```python
from build123d import *

# Parameters (mm, degrees)
SKETCH1_W                     = 96
SKETCH1_H                     = 96
SKETCH1_R                     = 13.97
BOSS_EXTRUDE1_DEPTH           = 5
FILLET1_R                     = 20
CBORE_FOR_M3_SHCS1_AT_2_COUNT = 2
CBORE_FOR_M3_SHCS1_AT_2_PITCH = 56.568542495
CBORE_FOR_M3_SHCS1_AT_3_COUNT = 2
CBORE_FOR_M3_SHCS1_AT_3_PITCH = 80
CBORE_FOR_M3_SHCS1_AT_4_COUNT = 2
CBORE_FOR_M3_SHCS1_AT_4_PITCH = 56.568542495
SKETCH7_R                     = 2
CUT_EXTRUDE1_DEPTH            = 69.066144301


with BuildPart() as part:
    # Sketch1 → Boss-Extrude1 (new body)
    with BuildSketch(Plane(origin=(0, 0, 0), x_dir=(1, 0, 0), z_dir=(0, 1, 0))):
        Rectangle(SKETCH1_W, SKETCH1_H)
        with Locations(Location((0, 0, 0), (0, 0, 270))):
            Circle(SKETCH1_R, mode=Mode.SUBTRACT)
    extrude(amount=BOSS_EXTRUDE1_DEPTH)

    # Fillet1
    fillet1_edges = [part.edges().sort_by_distance(p)[0] for p in [
        (-48, 2.5, -48),
        (48, 2.5, -48),
        (48, 2.5, 48),
        (-48, 2.5, 48),
    ]]
    fillet(fillet1_edges, radius=FILLET1_R)

    # Sketch6 → CBORE for M3 SHCS1 (revolve, cut)
    with BuildSketch(Plane(origin=(-40, 0, 0), x_dir=(0, 0, -1), z_dir=(1, 0, 0))):
        Polygon((0, 0), (0, 5), (1.7, 5), (1.7, 3), (3.25, 3), (3.25, 0.025), (3.275, 0), align=None)
    cbore_for_m3_shcs1 = revolve(axis=Axis((-40, -6.35, 0), (0, 1, 0)), mode=Mode.SUBTRACT)

    # CBORE for M3 SHCS1 at 2: CBORE for M3 SHCS1 ×2
    with Locations(*[Vector(0.7071067811865476, 0, 0.7071067811865476) * (i * CBORE_FOR_M3_SHCS1_AT_2_PITCH) for i in range(1, CBORE_FOR_M3_SHCS1_AT_2_COUNT)]):
        add(cbore_for_m3_shcs1, mode=Mode.SUBTRACT)

    # CBORE for M3 SHCS1 at 3: CBORE for M3 SHCS1 ×2
    with Locations(*[(i * CBORE_FOR_M3_SHCS1_AT_3_PITCH, 0, 0) for i in range(1, CBORE_FOR_M3_SHCS1_AT_3_COUNT)]):
        add(cbore_for_m3_shcs1, mode=Mode.SUBTRACT)

    # CBORE for M3 SHCS1 at 4: CBORE for M3 SHCS1 ×2
    with Locations(*[Vector(0.7071067811865476, 0, -0.7071067811865476) * (i * CBORE_FOR_M3_SHCS1_AT_4_PITCH) for i in range(1, CBORE_FOR_M3_SHCS1_AT_4_COUNT)]):
        add(cbore_for_m3_shcs1, mode=Mode.SUBTRACT)

    # Sketch7 → Cut-Extrude1 (cut, through all)
    with BuildSketch(Plane.XZ):
        with Locations(Location((-27.5, 0, 0), (0, 0, 270))):
            Circle(SKETCH7_R)
        with Locations(Location((0, 27.5, 0), (0, 0, 270))):
            Circle(SKETCH7_R)
        with Locations(Location((27.5, 0, 0), (0, 0, 270))):
            Circle(SKETCH7_R)
        with Locations(Location((0, -27.5, 0), (0, 0, 270))):
            Circle(SKETCH7_R)
    extrude(amount=-CUT_EXTRUDE1_DEPTH, mode=Mode.SUBTRACT)


solid = part.part
```
The model under review builds one solid part; all positions refer to its coordinate system, in mm. A direction names the side the tool comes from. Round coordinates to 2 decimals unless told otherwise and drop trailing zeros. Loops run counter-clockwise (first coordinate to the right, second up) from the corner with the lowest first, then second, coordinate; pieces in that order, holes last. Notation, with made-up numbers: M 28,62 L 51,62 A19 ccw 51,87 Z; hole C -5,38 d4. An arc over 180 degrees is marked long. Put each result on its own line as item: value.
Q1. Consider section A-A, the plane y = 1.7. Count the separate pieces of the cut face and the enclosed holes in it, then the cut area to 3 significant figures.
Result set:
separate pieces: 1
enclosed holes: 9
area: 8,080 mm²
Q2. Mouldability with a two-part tool opening along Z and no side actions: class faces 3 (the cylindrical face through (-0.766, 2.465, 25.653)), 4 (the flat face through (0, 2, -48)), 5 (the cylindrical face through (-42.297, 2.535, 41.986)) as released by +Z, released by -Z, zero draft, split by the parting line, or undercut.
Result set:
face 3: undercut
face 4: released by -Z
face 5: released by +Z
Q3. Consider section D-D, the plane x = -34.5. Give the boundary of the cut face in (y, z), then the cut area to 3 significant figures.
Result set:
outline: M 0,-46.91 L 5,-46.91 L 5,46.91 L 0,46.91 Z
area: 469 mm²
Q4. Consider section B-B, the plane z = -40. Give the boundary of the cut face in (x, y) (3 decimals), then the cut area to 3 significant figures.
Result set:
outline: M -44,0 L -3.275,0 L -3.25,0.025 L -3.25,3 L -1.7,3 L -1.7,5 L -44,5 Z; M 1.7,3 L 3.25,3 L 3.25,0.025 L 3.275,0 L 44,0 L 44,5 L 1.7,5 Z
area: 414 mm²
Q5. Machinability: for faces 1 (the flat face through (1.4, 3, -38.6)), 2 (the cylindrical face through (41.986, 2.535, 42.297)), which of the approach directions +Z, -Z, +X, -X, +Y, -Y give a long, thin tool a straight path to every point of the face, cutting with its end or side? Answer none if there is none.
Result set:
face 1: -Y
face 2: +Z, +X, +Y, -Y
Q6. To check wall thickness, follow L1, parallel to X at y = 4, z = 0; L2, parallel to Z at x = 40, y = 1; L3, parallel to X at y = 3, z = 27.5. State the ranges of each line that lie inside material, in increasing order.
Result set:
L1: x = -48 to -41.7, -38.3 to -29.5, -25.5 to -13.97, 13.97 to 25.5, 29.5 to 38.3, 41.7 to 48
L2: z = -44 to -3.25, 3.25 to 44
L3: x = -48 to -2, 2 to 48
Q7. For pin 1 (4 mm diameter, centred on x = 40, z = 0, fed in from -Y); pin 2 (3.5 mm diameter, centred on x = 0, z = 27.5, fed in from +Y), all flat-tipped, find the tip position at first contact; note any pin that passes through.
Result set:
pin 1: stops at y = 3
pin 2: passes through
